Source: three-view drawing plus pictorial views. Frame: mm from the lowest corner of the part. Give positions to 0.01 mm unless a question says otherwise; leave off trailing zeros. Loops run counter-clockwise (first coordinate to the right, second up) from the corner with the lowest first, then second, coordinate; pieces in that order, holes last. Notation, with made-up numbers: M 25,42 L 59,42 A24 cw 59,64 Z; hole C 42.25,54.25 d4. An arc over 180 degrees is marked long. Answer as a JSON object with one key per item and string values. Group by question number.
1) Draft query along Z for the marked faces 1, 2 and 3. Return one class per face: +Z half, -Z half, draft (parallel to the pull), parting line (faces both ways), or undercut.
2) Section query C-C on y = 108. Return loops of the section in (x, z).
3) Section query A-A on z = 59.5. Return loops of the section in (x, y).
4) Section query B-B on x = 59.5. Return loops of the section in (y, z).
5) Ray query, L1, parallel to X at y = 49.5, z = 24 (1 decimal); L2, parallel to Z at x = 66, y = 111 (1 decimal); L3, parallel to Z at x = 78, y = 12 (1 decimal). Return the intervals inside material, ascending.
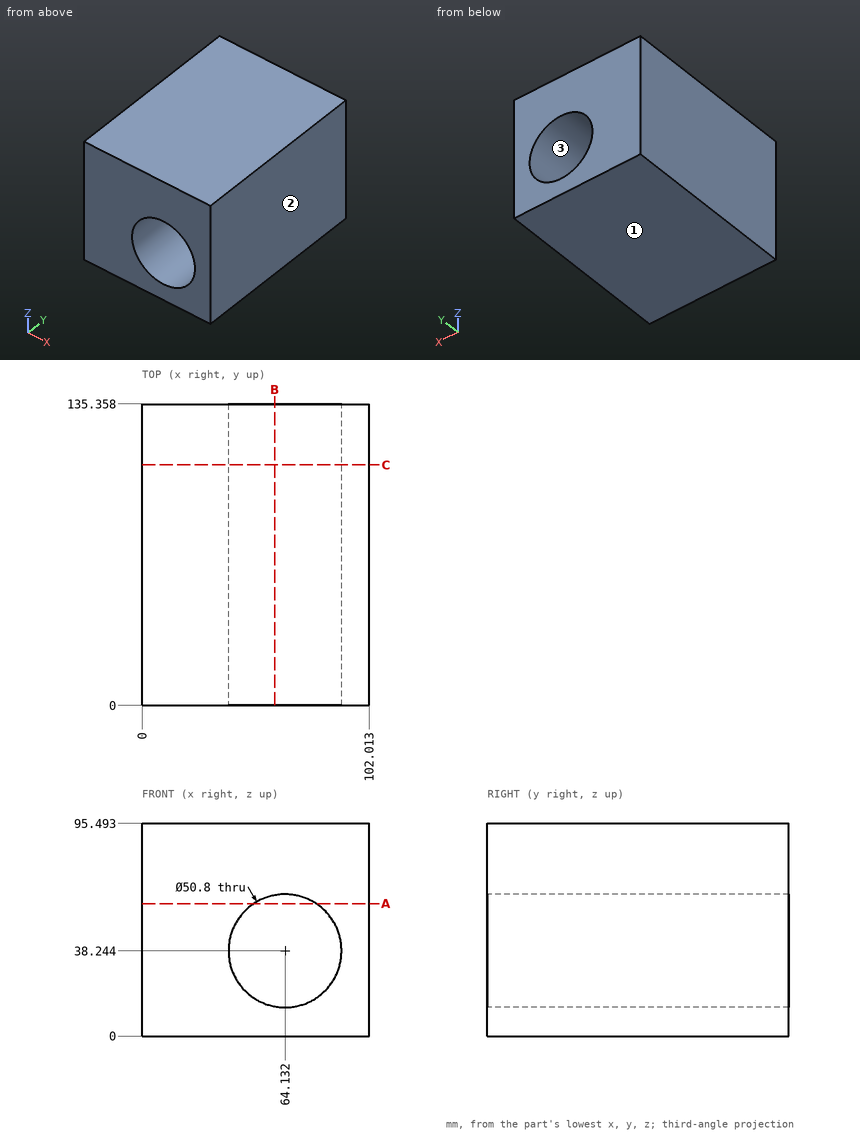
Output:
{
 "1": {"face 1": "-Z half", "face 2": "draft", "face 3": "undercut"},
 "2": {"outline": "M 0,0 L 102.01,0 L 102.01,95.49 L 0,95.49 Z; hole C 64.13,38.24 d50.8"},
 "3": {"outline": "M 0,0 L 50.23,0 L 50.23,135.36 L 0,135.36 Z; M 78.04,0 L 102.01,0 L 102.01,135.36 L 78.04,135.36 Z"},
 "4": {"outline": "M 0,0 L 135.36,0 L 135.36,13.27 L 0,13.27 Z; M 0,63.22 L 135.36,63.22 L 135.36,95.49 L 0,95.49 Z"},
 "5": {"L1": "x = 0 to 43.1, 85.2 to 102", "L2": "z = 0 to 12.9, 63.6 to 95.5", "L3": "z = 0 to 17, 59.5 to 95.5"}
}
